CAD build for the part. Positions are in the model's coordinates, mm. A direction names the side the tool comes from. Coordinates: 2 decimals unless noted, no trailing zeros. Loops run counter-clockwise (first coordinate to the right, second up) from the corner with the lowest first, then second, coordinate; pieces in that order, holes last. Notation, with made-up numbers: (79.5, 72) -> (99.5, 72) arc R17 ccw to (99.5, 105) -> close; hole circle Ø9 at (60.25, 30.5). An arc over 180 degrees is marked (long way). Write each question's results on one line, items separated by ' | '.
```python
from build123d import *

# Parameters (mm, degrees)
F1_DEPTH = 1000


with BuildPart() as f1:
    # F0 (on Right) → F1 (new body)
    with BuildSketch(Plane.YZ):
        with BuildLine():
            Line((56.45, 0), (56.45, 12.5))
            Line((56.45, 12.5), (62.052685, 14.539211))
            ThreePointArc((62.052685, 14.539211), (63.499961, 24.447472), (62.082432, 34.360032))
            ThreePointArc((62.082432, 34.360032), (31.75, 41.5), (1.417568, 34.360032))
            ThreePointArc((1.417568, 34.360032), (3.9e-05, 24.447472), (1.447315, 14.539211))
            Line((1.447315, 14.539211), (7.05, 12.5))
            Line((7.05, 12.5), (7.05, 0))
            Line((7.05, 0), (8.85, 0))
            Line((8.85, 0), (8.85, 2))
            Line((8.85, 2), (10.91777, 2))
            ThreePointArc((10.91777, 2), (12.319719, 3.861416), (13.495637, 5.873267))
            ThreePointArc((13.495637, 5.873267), (13.476243, 6.361375), (13.05, 6.6))
            Line((13.05, 6.6), (8.85, 6.6))
            Line((8.85, 6.6), (8.85, 13.760374))
            Line((8.85, 13.760374), (2.929064, 15.915418))
            ThreePointArc((2.929064, 15.915418), (1.800001, 24.507341), (2.932863, 33.098764))
            ThreePointArc((2.932863, 33.098764), (31.75, 39.7), (60.567137, 33.098764))
            ThreePointArc((60.567137, 33.098764), (61.699999, 24.507341), (60.570936, 15.915418))
            Line((60.570936, 15.915418), (54.65, 13.760374))
            Line((54.65, 13.760374), (54.65, 6.6))
            Line((54.65, 6.6), (50.45, 6.6))
            ThreePointArc((50.45, 6.6), (50.023757, 6.361375), (50.004363, 5.873267))
            ThreePointArc((50.004363, 5.873267), (51.180281, 3.861416), (52.58223, 2))
            Line((52.58223, 2), (54.65, 2))
            Line((54.65, 2), (54.65, 0))
            Line((54.65, 0), (56.45, 0))
        make_face()
    extrude(amount=F1_DEPTH)


solid = f1.part
```
Q1. Cut at A-A on x = 463.5. Write the cut outline in (y, z).
Results are:
outline: (1.42, 34.36) arc R35 ccw to (1.45, 14.54) -> (7.05, 12.5) -> (7.05, 0) -> (8.85, 0) -> (8.85, 2) -> (10.92, 2) arc R20 ccw to (13.5, 5.87) arc R0.5 ccw to (13.05, 6.6) -> (8.85, 6.6) -> (8.85, 13.76) -> (2.93, 15.92) arc R33.2 cw to (2.93, 33.1) arc R66.2 cw to (60.57, 33.1) arc R33.2 cw to (60.57, 15.92) -> (54.65, 13.76) -> (54.65, 6.6) -> (50.45, 6.6) arc R0.5 ccw to (50, 5.87) arc R20 ccw to (52.58, 2) -> (54.65, 2) -> (54.65, 0) -> (56.45, 0) -> (56.45, 12.5) -> (62.05, 14.54) arc R35 ccw to (62.08, 34.36) arc R68 ccw to start
Q2. Wall check: L1, parallel to Y at x = 391, z = 25; L2, parallel to Y at x = 883, z = 22; L3, parallel to Z at x = 829.5, y = 55.5. Give the ranges that are in metal, low to high. Write a range as from..to.
Results are:
L1: 0..1.8, 61.7..63.5 | L2: 0.09..1.89, 61.61..63.41 | L3: 0..14.07, 35.29..37.22
Q3. Which spindle directions (+Z, -Z, +X, -X, +Y, -Y) get a long thin tool onto all of the face, cutting with end or side? Do faces 1 (the cylindrical face through (493, 61.7, 24.6)), 2 (the cylindrical face through (493, 63.5, 24.3)). Say none if no direction does.
Results are:
face 1: +X, -X | face 2: +X, -X, +Y
Q4. Drop flat-ended pins along their axis: pin 1 (2 mm diameter, centred on x = 286, y = 10.5, fed in from +Z); pin 2 (1 mm diameter, centred on x = 117.5, y = 32.5, fed in from -Z); pin 3 (0.6 mm diameter, centred on x = 374, z = 1.5, fed in from -Y); pin 4 (12 mm diameter, centred on y = 45.5, z = 30.5, fed in from +X). Give the stop position or say it passes through.
Results are:
pin 1: z = 38.41 | pin 2: z = 39.69 | pin 3: y = 7.05 | pin 4: through
Q5. Pull direction Z, two halves, no side cores. Call faces 3 (the flat face through (0, 32, 41)), 4 (the cylindrical face through (493, 0, 24.6)), 5 (the cylindrical face through (493, 32.2, 41.5)), 6 (the cylindrical face through (493, 1.8, 24.4)): +Z half, -Z half, draft (parallel to the pull), parting line (faces both ways), or undercut.
Results are:
face 3: draft | face 4: parting line | face 5: +Z half | face 6: undercut
Q6. Cut at B-B on y = 31.5. Write the cut outline in (x, z), and give its area (3 significant figures).
Results are:
outline: (0, 39.7) -> (1000, 39.7) -> (1000, 41.5) -> (0, 41.5) -> close | area: 1,800 mm^2
